The model under review builds one solid part; all positions refer to its coordinate system, in mm. A direction names the side the tool comes from. Coordinates: 2 decimals unless noted, no trailing zeros. Write each loop counter-clockwise with the first axis right and the second up, starting at its lowest first coordinate (ties: lowest second). Pieces come first, ordered by that corner, then holes.
1) Add section A-A, the plane x = -37. State the section outline as (y, z) points.
2) Add section D-D, the plane z = 4. State the section outline as (x, y) points.
3) For line 1 (Y direction, x = -44.5, z = 12.5); line 2 (Y direction, x = -13, z = 10); line 3 (Z direction, x = -30.5, y = 51.5), list the stretches that pass through material, from the lowest coordinate up.
4) Mouldability with a two-part tool opening along Y and no side actions: class faces 1 (the flat face through (-93.94, 43.242, 9.015)), 2 (the cylindrical face through (8.935, 39.92, 12.325)), 3 (the cylindrical face through (-5.36, -25.93, 12.32)) as released by +Y, released by -Y, zero draft, split by the parting line, or undercut.
5) For P1, Ø2, axis at x = -19.5, z = 21.5, coming from the -Y side; P2, Ø6.5, axis at x = -95, z = 14.5, coming from the -Y side; P3, Ø5, axis at y = 6, z = 21.5, coming from the -X side, all flat-tipped, find the tip position at first contact; note any pin that passes through.
6) Add section C-C, the plane y = -44.5. State the section outline as (x, z) points.
7) Machinability: for faces 4 (the flat face through (-67.34, 47.17, -6.75)), 5 (the flat face through (-98.16, 43.44, 16.2)), 6 (the flat face through (-78.058, -55, 12)), 7 (the cylindrical face through (-24.893, -42.573, 14.127)), which of the approach directions +Z, -Z, +X, -X, +Y, -Y give a long, thin tool a straight path to every point of the face, cutting with its end or side? Answer none if there is none.
8) Add section B-B, the plane x = -11. State the section outline as (y, z) points.
from build123d import *

# Parameters (mm, degrees)
SKETCH1_W                = 15
SKETCH1_H                = 20
BOSS_EXTRUDE2_DEPTH      = 25
BOSS_EXTRUDE4_DEPTH      = 20
SKETCH2_R                = 15
BOSS_EXTRUDE5_DEPTH      = 46
BOSS_EXTRUDE5_DEPTH_BACK = 54
SKETCH5_R                = 12.5
CUT_EXTRUDE1_DEPTH       = 95
SKETCH6_R                = 3
CUT_EXTRUDE2_DEPTH       = 24
CUT_EXTRUDE3_DEPTH       = 41.001633849
CUT_EXTRUDE3_DEPTH_BACK  = 16.100391206
CUT_EXTRUDE5_DEPTH       = 24
SKETCH11_R               = 2.435
CUT_EXTRUDE6_DEPTH       = 104.651176362
CUT_EXTRUDE7_START       = -12
CUT_EXTRUDE7_DEPTH       = 10


with BuildPart() as part:
    # Sketch1 → Boss-Extrude2 (new body)
    with BuildSketch(Plane.XY):
        with BuildLine():
            ThreePointArc((5.591494761, 0), (-5.652702459, -26.223247911), (-32.057903297, -37.033246562))
            Line((-32.057903297, -37.033246562), (-32.057903297, -57.033246562))
            ThreePointArc((-32.057903297, -57.033246562), (8.489751808, -40.365693604), (25.593272966, 0))
            ThreePointArc((25.593272966, 0), (8.489751808, 40.365693604), (-32.057903297, 57.033246562))
            Line((-32.057903297, 57.033246562), (-32.057903297, 37.033246562))
            ThreePointArc((-32.057903297, 37.033246562), (-5.652702459, 26.223247911), (5.591494761, 0))
        make_face()
        with Locations((-39.557903297, 47.033246562)):
            Rectangle(SKETCH1_W, SKETCH1_H)
    extrude(amount=BOSS_EXTRUDE2_DEPTH)

    # Sketch3 → Boss-Extrude4 (add)
    with BuildSketch(Plane(origin=(0, 57.033246562, 0), x_dir=(1, 0, 0), z_dir=(0, 1, 0))):
        with BuildLine():
            Line((-47.057903297, -24.901242643), (-47.057903297, 0))
            Line((-47.057903297, 0), (-88.188861039, 13.690366027))
            ThreePointArc((-88.188861039, 13.690366027), (-124.440854646, -12.450621321), (-88.188861039, -38.591608669))
            Line((-88.188861039, -38.591608669), (-47.057903297, -24.901242643))
        make_face()
    extrude(amount=-BOSS_EXTRUDE4_DEPTH)

    # Sketch2 → Boss-Extrude5 (add, two sides)
    with BuildSketch(Plane.ZY.offset(32.057903297)) as boss_extrude5_sk:
        with Locations((12.5, -54.966753438)):
            Circle(SKETCH2_R)
    extrude(amount=BOSS_EXTRUDE5_DEPTH)
    extrude(boss_extrude5_sk.sketch, amount=-BOSS_EXTRUDE5_DEPTH_BACK)

    # Sketch5 → Cut-Extrude1 (cut)
    with BuildSketch(Plane(origin=(21.942096703, 0, 0), x_dir=(0, 0, -1), z_dir=(1, 0, 0))):
        with Locations((-12.5, -54.966753438)):
            Circle(SKETCH5_R)
    extrude(amount=-CUT_EXTRUDE1_DEPTH, mode=Mode.SUBTRACT)

    # Sketch6 → Cut-Extrude2 (cut)
    with BuildSketch(Plane(origin=(0, 57.033246562, 0), x_dir=(1, 0, 0), z_dir=(0, 1, 0))):
        with Locations((-96.052193002, -12.606102104)):
            Circle(SKETCH6_R)
    extrude(amount=-CUT_EXTRUDE2_DEPTH, mode=Mode.SUBTRACT)

    # Sketch7 → Cut-Extrude3 (cut, two sides)
    with BuildSketch(Plane.XY) as cut_extrude3_sk:
        Polygon((-124.440854646, 44.571784262), (-47.057903297, 37.033246562), (-124.440854646, 37.033246562), align=None)
    extrude(amount=CUT_EXTRUDE3_DEPTH, mode=Mode.SUBTRACT)
    extrude(cut_extrude3_sk.sketch, amount=-CUT_EXTRUDE3_DEPTH_BACK, mode=Mode.SUBTRACT)

    # Sketch5_3 → Cut-Extrude5 (cut)
    with BuildSketch(Plane(origin=(21.942096703, 0, 0), x_dir=(0, 0, -1), z_dir=(1, 0, 0))):
        with BuildLine():
            Line((2.5, -54.966753438), (0, -54.966753438))
            ThreePointArc((0, -54.966753438), (-12.5, -67.466753438), (-25, -54.966753438))
            Line((-25, -54.966753438), (-27.5, -54.966753438))
            ThreePointArc((-27.5, -54.966753438), (-12.5, -69.966753438), (2.5, -54.966753438))
        make_face()
    extrude(amount=-CUT_EXTRUDE5_DEPTH, mode=Mode.SUBTRACT)

    # Sketch11 → Cut-Extrude6 (cut, through all)
    with BuildSketch(Plane.ZY.offset(78.057903297)):
        with Locations((14.672182151, -59.168482213)):
            Circle(SKETCH11_R)
    extrude(amount=-CUT_EXTRUDE6_DEPTH, mode=Mode.SUBTRACT)

    # Sketch13 → Cut-Extrude7 (cut)
    with BuildSketch(Plane(origin=(0, 57.033246562, 0), x_dir=(1, 0, 0), z_dir=(0, 1, 0)).offset(CUT_EXTRUDE7_START)):
        Polygon((-96.052193002, -7.794849861), (-100.218859669, -10.200475983), (-100.218859669, -15.011728226), (-96.052193002, -17.417354348), (-91.885526335, -15.011728226), (-91.885526335, -10.200475983), align=None)
    extrude(amount=-CUT_EXTRUDE7_DEPTH, mode=Mode.SUBTRACT)


solid = part.part
Geometry results:
1. outline: circle Ø30 at (-54.97, 12.5); (37.03, 0) - (57.03, 0) - (57.03, 25) - (37.03, 25) - close; hole circle Ø25 at (-54.97, 12.5)
2. outline: (-123.11, 44.44) - (-47.06, 37.03) - (-32.06, 37.03) arc R37.65 cw to (5.59, 0) arc R37.65 cw to (-32.06, -37.03) - (-32.06, -42.61) - (-78.06, -42.61) - (-78.06, -67.33) - (-2.06, -67.33) - (-2.06, -64.13) - (-73.06, -64.13) - (-73.06, -45.8) - (21.94, -45.8) - (21.94, -42.61) - (6.09, -42.61) arc R57.65 ccw to (25.59, 0) arc R57.65 ccw to (-32.06, 57.03) - (-123.11, 57.03) - close
3. line 1: y = -69.97 to -67.47, -42.47 to -39.97, 37.03 to 57.03
3. line 2: y = -69.76 to -67.21, -42.72 to -31.85, 31.85 to 53.79
3. line 3: z = 0 to 25
4. face 1: zero draft
4. face 2: released by +Y
4. face 3: undercut
5. P1: stops at y = -67.66
5. P2: stops at y = 41.39
5. P3: stops at x = 4.48
6. outline: (-78.06, 1.76) - (-32.06, 1.76) - (-32.06, 0) - (3.83, 0) - (3.83, 1.76) - (21.94, 1.76) - (21.94, 5.67) - (-73.06, 5.67) - (-73.06, 19.33) - (21.94, 19.33) - (21.94, 23.24) - (3.83, 23.24) - (3.83, 25) - (-32.06, 25) - (-32.06, 23.24) - (-78.06, 23.24) - close
7. face 4: -Z, +X, +Y
7. face 5: -Y
7. face 6: +Z, -Z, -X, -Y
7. face 7: +X
8. outline: (-46.68, 0) - (-30.59, 0) - (-30.59, 25) - (-46.68, 25) arc R15 ccw (long way) to start; (30.59, 0) - (53.05, 0) - (53.05, 25) - (30.59, 25) - close; hole circle Ø25 at (-54.97, 12.5)
